Geometry: final body of the model. Coordinates: model frame, mm. Give positions to 0.01 mm unless a question says otherwise; leave off trailing zeros. Loops run counter-clockwise (first coordinate to the right, second up) from the corner with the lowest first, then second, coordinate; pieces in that order, holes last. Notation, with made-up numbers: (89, 1) -> (140, 1) arc R24 cw to (140, 30) -> close; hole circle Ø10 at (-16.5, 57.5). An arc over 180 degrees is marked (long way). Answer in a Markdown table with one row per item. Add a question column.
1) Section query C-C (y = -8). Return the cut outline in (x, z).
2) Section query B-B (z = 0.8). Return the cut outline in (x, y).
3) Line query: line 1 (X direction, y = -0.25, z = 1.8); line 2 (Y direction, x = -75, z = 1.95); line 3 (X direction, y = -1, z = 0.6). Output: solid intervals per line, ascending. Write a range as from..to.
4) Draft query along X for faces 1 (the cylindrical face through (-85, 0, 1)), 2 (the cylindrical face through (-77.4, -1.8, 1.5)), 3 (the flat face through (1, 10, 1)), 4 (the cylindrical face through (72.6, -1.8, 1.5)). Return one class per face: +X half, -X half, draft (parallel to the pull), parting line (faces both ways), or undercut.
5) First-contact query: P1, Ø7, axis at x = 75, y = 0, coming from the -Z side; P2, Ø1, axis at y = -6.5, z = 2.5, coming from the +X side. Flat tips, straight axial feed; report the tip coordinate or a pass-through.
6) Section query A-A (y = 0). Return the cut outline in (x, z), plus the area to 3 significant figures.
```python
from build123d import *

# Parameters (mm, degrees)
SKETCH1_R           = 3
BOSS_EXTRUDE1_DEPTH = 3


with BuildPart() as part:
    # Sketch1 → Boss-Extrude1 (new body)
    with BuildSketch(Plane.XY):
        with BuildLine():
            Line((-75, -10), (75, -10))
            ThreePointArc((75, -10), (85, 0), (75, 10))
            Line((75, 10), (-75, 10))
            ThreePointArc((-75, 10), (-85, 0), (-75, -10))
        make_face()
        with Locations((-75, 0)):
            Circle(SKETCH1_R, mode=Mode.SUBTRACT)
        with BuildLine():
            ThreePointArc((-16.4, -1.6), (-17.2, 0), (-16.4, 1.6))
            Line((-16.4, 1.6), (-16.4, 6.2))
            Line((-16.4, 6.2), (6.2, 6.2))
            Line((6.2, 6.2), (6.2, 2.64368992))
            Line((6.2, 2.64368992), (15.34156858, 1.994983292))
            ThreePointArc((15.34156858, 1.994983292), (17.2, 0), (15.34156858, -1.994983292))
            Line((15.34156858, -1.994983292), (6.2, -2.64368992))
            Line((6.2, -2.64368992), (6.2, -6.2))
            Line((6.2, -6.2), (-16.4, -6.2))
            Line((-16.4, -6.2), (-16.4, -1.6))
        make_face(mode=Mode.SUBTRACT)
        with Locations((75, 0)):
            Circle(SKETCH1_R, mode=Mode.SUBTRACT)
        with BuildLine():
            Line((-15.34156858, 1.994983292), (-1.88348082, 2.95))
            ThreePointArc((-1.88348082, 2.95), (0, 3.5), (1.88348082, 2.95))
            Line((1.88348082, 2.95), (6.2, 2.64368992))
            Line((6.2, 2.64368992), (6.2, 6.2))
            Line((6.2, 6.2), (-16.4, 6.2))
            Line((-16.4, 6.2), (-16.4, 1.6))
            ThreePointArc((-16.4, 1.6), (-15.899252826, 1.873778398), (-15.34156858, 1.994983292))
        make_face()
        with BuildLine():
            ThreePointArc((-15.34156858, -1.994983292), (-15.899252826, -1.873778398), (-16.4, -1.6))
            Line((-16.4, -1.6), (-16.4, -6.2))
            Line((-16.4, -6.2), (6.2, -6.2))
            Line((6.2, -6.2), (6.2, -2.64368992))
            Line((6.2, -2.64368992), (1.88348082, -2.95))
            ThreePointArc((1.88348082, -2.95), (0, -3.5), (-1.88348082, -2.95))
            Line((-1.88348082, -2.95), (-15.34156858, -1.994983292))
        make_face()
        with BuildLine():
            ThreePointArc((1.88348082, 2.95), (0, 3.5), (-1.88348082, 2.95))
            Line((-1.88348082, 2.95), (-15.34156858, 1.994983292))
            ThreePointArc((-15.34156858, 1.994983292), (-15.899252826, 1.873778398), (-16.4, 1.6))
            Line((-16.4, 1.6), (-16.4, -1.6))
            ThreePointArc((-16.4, -1.6), (-15.899252826, -1.873778398), (-15.34156858, -1.994983292))
            Line((-15.34156858, -1.994983292), (-1.88348082, -2.95))
            ThreePointArc((-1.88348082, -2.95), (0, -3.5), (1.88348082, -2.95))
            Line((1.88348082, -2.95), (6.2, -2.64368992))
            Line((6.2, -2.64368992), (6.2, 2.64368992))
            Line((6.2, 2.64368992), (1.88348082, 2.95))
        make_face()
        with BuildLine():
            Line((-16.4, -1.6), (-16.4, 1.6))
            ThreePointArc((-16.4, 1.6), (-17.2, 0), (-16.4, -1.6))
        make_face()
        with BuildLine():
            Line((15.34156858, 1.994983292), (6.2, 2.64368992))
            Line((6.2, 2.64368992), (6.2, -2.64368992))
            Line((6.2, -2.64368992), (15.34156858, -1.994983292))
            ThreePointArc((15.34156858, -1.994983292), (17.2, 0), (15.34156858, 1.994983292))
        make_face()
    extrude(amount=BOSS_EXTRUDE1_DEPTH)


solid = part.part
```
Evaluation:
| question | item | result |
|---|---|---|
| 1 | outline | (-81, 0) -> (81, 0) -> (81, 3) -> (-81, 3) -> close |
| 2 | outline | (-75, -10) -> (75, -10) arc R10 ccw to (75, 10) -> (-75, 10) arc R10 ccw to start; hole circle Ø6 at (-75, 0); hole circle Ø6 at (75, 0) |
| 3 | line 1 | -85..-77.99, -72.01..72.01, 77.99..85 |
| 3 | line 2 | -10..-3, 3..10 |
| 3 | line 3 | -84.95..-77.83, -72.17..72.17, 77.83..84.95 |
| 4 | face 1 | -X half |
| 4 | face 2 | undercut |
| 4 | face 3 | draft |
| 4 | face 4 | undercut |
| 5 | P1 | z = 0 |
| 5 | P2 | x = 83 |
| 6 | outline | (-85, 0) -> (-78, 0) -> (-78, 3) -> (-85, 3) -> close; (-72, 0) -> (72, 0) -> (72, 3) -> (-72, 3) -> close; (78, 0) -> (85, 0) -> (85, 3) -> (78, 3) -> close |
| 6 | area | 474 mm² |
